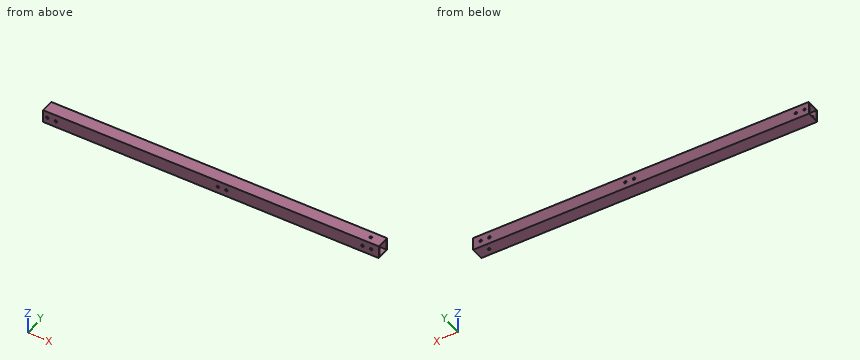
from build123d import *

# Parameters (mm, degrees)
SKETCH_1_W          = 15
SKETCH_1_H          = 15
SKETCH_1_W_2        = 13
SKETCH_1_H_2        = 13
EXTRUDE_1_DEPTH     = 390
SKETCH_2_R          = 1.45
CUT_EXTRUDE_1_DEPTH = 391.36041039
SKETCH_3_R          = 1.45
CUT_EXTRUDE_2_DEPTH = 391.36041039


with BuildPart() as part:
    # 草图1 → 凸台-拉伸1 (new body)
    with BuildSketch(Plane(origin=(0, 0, 0), x_dir=(0, 0, -1), z_dir=(1, 0, 0))):
        Rectangle(SKETCH_1_W, SKETCH_1_H)
        Rectangle(SKETCH_1_W_2, SKETCH_1_H_2, mode=Mode.SUBTRACT)
    extrude(amount=EXTRUDE_1_DEPTH)

    # 草图2 → 切除-拉伸1 (cut, through all)
    with BuildSketch(Plane(origin=(0, 7.5, 0), x_dir=(1, 0, 0), z_dir=(0, 1, 0))):
        with Locations(Location((203, 0, 0), (0, 0, 270))):
            Circle(SKETCH_2_R)
        with Locations(Location((213, 0, 0), (0, 0, 270))):
            Circle(SKETCH_2_R)
        with Locations(Location((15, 0, 0), (0, 0, 270))):
            Circle(SKETCH_2_R)
        with Locations(Location((5, 0, 0), (0, 0, 270))):
            Circle(SKETCH_2_R)
        with Locations(Location((381, 0, 0), (0, 0, 270))):
            Circle(SKETCH_2_R)
        with Locations(Location((371, 0, 0), (0, 0, 270))):
            Circle(SKETCH_2_R)
    extrude(amount=-CUT_EXTRUDE_1_DEPTH, mode=Mode.SUBTRACT)

    # 草图3 → 切除-拉伸2 (cut, through all)
    with BuildSketch(Plane(origin=(0, 0, -7.5), x_dir=(-1, 0, 0), z_dir=(0, 0, -1))):
        with Locations((-376, 0)):
            Circle(SKETCH_3_R)
    extrude(amount=-CUT_EXTRUDE_2_DEPTH, mode=Mode.SUBTRACT)


solid = part.part
Read the model definition and answer for the solid it produces. Units are mm, in the model's axes. Give positions to 0.01 mm unless a question says otherwise; leave off trailing zeros. Write each loop counter-clockwise with the first axis right and the second up, starting at its lowest first coordinate (ties: lowest second). Pieces come first, ordered by that corner, then holes. Notation, with made-up numbers: (81, 3) - (129, 3) arc R21 cw to (129, 9) - close; hole circle Ø8 at (19, 74.25). An arc over 180 degrees is marked (long way). Answer in a Markdown table with one row per item. Add a question column.
Item 1: Section B-B, the plane x = 80.5 is taken. Write down the section's boundary in (y, z), and give its area (3 significant figures).
Item 2: Section A-A, the plane z = 4.25 is taken. Write down the section's boundary in (x, y).
Item 3: Find the intervals of material crossed by L1, parallel to Y at x = 87.5, z = -0.5; L2, parallel to Z at x = 203, y = 7.25, in increasing order.
Item 4: Flat-ended cylindrical pins translate along their axes: P1, Ø4, axis at y = 3, z = -0.5, coming from the +X side; P2, Ø3.5, axis at x = 371, z = 0, coming from the -Y side. Find the tip coordinate at first contact, or state that the pin passes through.
Recorded:
| question | item | result |
|---|---|---|
| 1 | outline | (-7.5, -7.5) - (7.5, -7.5) - (7.5, 7.5) - (-7.5, 7.5) - close; hole (-6.5, -6.5) - (6.5, -6.5) - (6.5, 6.5) - (-6.5, 6.5) - close |
| 1 | area | 56.0 mm2 |
| 2 | outline | (0, -7.5) - (390, -7.5) - (390, -6.5) - (0, -6.5) - close; (0, 6.5) - (390, 6.5) - (390, 7.5) - (0, 7.5) - close |
| 3 | L1 | y = -7.5 to -6.5, 6.5 to 7.5 |
| 3 | L2 | z = -7.5 to -1.45, 1.45 to 7.5 |
| 4 | P1 | passes through |
| 4 | P2 | stops at y = -7.5 |
